Could you check a few things on this model? Use its own coordinates, in mm. A direction names the side the tool comes from. Coordinates: 2 decimals unless noted, no trailing zeros. Order: outer loops, then holes, each group sorted by start corner. A loop starts at its lowest first (then second) coordinate and runs counter-clockwise, first axis right, second up. Notation, with made-up numbers: (75.5, 87) - (123.5, 87) arc R24 ccw to (123.5, 109) - close; hole circle Ø1 at (44, 76). An arc over 180 degrees is marked (long way). Answer as a JSON object with one key per item and string values. Group by question number.
(1) We'd pull the mould along Z, two halves only. Please class faces 5 (the cylindrical face through (-0.1, -2.9, 14.5)), 6 (the flat face through (-13, -22.5, 13)), 7 (the flat face through (-8, 1, 0)): pulls with the +Z half, pulls with the -Z half, needs draft (parallel to the pull), parting line crosses it, or undercut.
(2) Will these pins go through, and if not, where does the flat tip stop? P1, Ø12, axis at x = 0, y = 30, coming from the -Z side; P2, Ø1.5, axis at y = -33, z = 14.5, coming from the -X side; P3, Ø5, axis at y = 8, z = 15.5, coming from the +X side; P4, Ø2.5, axis at x = -13.5, z = 14.5, coming from the +Y side.
(3) Imagine slicing it at B-B, the plane x = -0.75. Write out the boundary of the cut face in (y, z).
(4) Which directions (+Z, -Z, +X, -X, +Y, -Y) give clear straight access to the entire face, cutting with the end or side of a thin tool? Please do faces 1 (the flat face through (-13, 2.5, 13)), 2 (the cylindrical face through (-0.1, -2.9, 11.5)), 3 (the flat face through (6.5, -3, 7)), 4 (the cylindrical face through (-0.1, -3.1, 23.5)).
(5) Imagine slicing it at D-D, the plane z = 3.75. Write out the boundary of the cut face in (x, y).
(6) Imagine slicing it at A-A, the plane z = 13. Write out the boundary of the cut face in (x, y), and give its area (3 significant figures).
(7) Imagine slicing it at C-C, the plane y = 34. Write out the boundary of the cut face in (x, z).
(8) Please list where these lines run through material, in increasing order: probe 1 along Y at (x, z) = (0, 12.75); probe 2 along Y at (x, z) = (0, 6.5); probe 3 along Y at (x, z) = (7, 7.25).
from build123d import *

# Parameters (mm, degrees)
ESBO_O1_R                = 7.65
RESSALTO_EXTRUS_O1_DEPTH = 26
RESSALTO_EXTRUS_O2_DEPTH = 13
ESBO_O7_W                = 15
ESBO_O7_H                = 25
RESSALTO_EXTRUS_O3_DEPTH = 3
ESBO_O8_R                = 1.5
CORTE_EXTRUS_O1_DEPTH    = 15


with BuildPart() as part:
    # Esbo_o1 → Ressalto-extrus_o1 (new body)
    with BuildSketch(Plane.XY):
        with BuildLine():
            Line((-11.65, 30), (-11.65, 28))
            Line((-11.65, 28), (-11.65, -30))
            ThreePointArc((-11.65, -30), (10.282205503, -35.477111465), (-6.5, -20.331882293))
            Line((-6.5, -20.331882293), (-6.5, 20.331882293))
            ThreePointArc((-6.5, 20.331882293), (10.282205503, 35.477111465), (-11.65, 30))
        make_face()
        with Locations(Location((0, 30, 0), (0, 0, 180))):
            Circle(ESBO_O1_R, mode=Mode.SUBTRACT)
        with Locations(Location((0, -30, 0), (0, 0, 180))):
            Circle(ESBO_O1_R, mode=Mode.SUBTRACT)
    extrude(amount=RESSALTO_EXTRUS_O1_DEPTH)

    # Esbo_o6 → Ressalto-extrus_o2 (add)
    with BuildSketch(Plane(origin=(-6.5, 0, 0), x_dir=(0, 0, -1), z_dir=(1, 0, 0))):
        with BuildLine():
            Line((-17.5, -6), (-20.5, -6))
            ThreePointArc((-20.5, -6), (-23.5, -3), (-20.5, 0))
            Line((-20.5, 0), (-17.5, 0))
            ThreePointArc((-17.5, 0), (-14.5, -3), (-17.5, -6))
        make_face()
        with BuildLine():
            Line((-8.5, -6), (-5.5, -6))
            ThreePointArc((-5.5, -6), (-2.5, -3), (-5.5, 0))
            Line((-5.5, 0), (-8.5, 0))
            ThreePointArc((-8.5, 0), (-11.5, -3), (-8.5, -6))
        make_face()
    extrude(amount=RESSALTO_EXTRUS_O2_DEPTH)

    # Esbo_o7 → Ressalto-extrus_o3 (add)
    with BuildSketch(Plane.ZY.offset(11.65)):
        with Locations((13, -10)):
            Rectangle(ESBO_O7_W, ESBO_O7_H)
    extrude(amount=RESSALTO_EXTRUS_O3_DEPTH)

    # Esbo_o8 → Corte-extrus_o1 (cut)
    with BuildSketch(Plane.ZY.offset(14.65)):
        with Locations(Location((13, -10, 0), (0, 0, 270))):
            Circle(ESBO_O8_R)
    extrude(amount=-CORTE_EXTRUS_O1_DEPTH, mode=Mode.SUBTRACT)


solid = part.part
Result set:
{
 "1": {"face 5": "undercut", "face 6": "needs draft", "face 7": "pulls with the -Z half"},
 "2": {"P1": "passes through", "P2": "stops at x = -11.43", "P3": "stops at x = -6.5", "P4": "stops at y = 2.5"},
 "3": {"outline": "(-41.63, 0) - (-37.61, 0) - (-37.61, 26) - (-41.63, 26) - close; (-22.39, 0) - (-18.37, 0) - (-18.37, 26) - (-22.39, 26) - close; (-6, 5.5) arc R3 ccw to (0, 5.5) - (0, 8.5) arc R3 ccw to (-6, 8.5) - close; (-6, 17.5) arc R3 ccw to (0, 17.5) - (0, 20.5) arc R3 ccw to (-6, 20.5) - close; (18.37, 0) - (22.39, 0) - (22.39, 26) - (18.37, 26) - close; (37.61, 0) - (41.63, 0) - (41.63, 26) - (37.61, 26) - close"},
 "4": {"face 1": "+Z, -Z, -X, +Y", "face 2": "+X", "face 3": "+Z, -Z, +X", "face 4": "+Z, +X"},
 "5": {"outline": "(-11.65, -30) arc R11.65 ccw (long way) to (-6.5, -20.33) - (-6.5, -5.44) - (6.5, -5.44) - (6.5, -0.56) - (-6.5, -0.56) - (-6.5, 20.33) arc R11.65 ccw (long way) to (-11.65, 30) - close; hole circle Ø15.3 at (0, -30); hole circle Ø15.3 at (0, 30)"},
 "6": {"outline": "(-14.65, -22.5) - (-11.65, -22.5) - (-11.65, -30) arc R11.65 ccw (long way) to (-6.5, -20.33) - (-6.5, -11.5) - (-14.65, -11.5) - close; (-14.65, -8.5) - (-6.5, -8.5) - (-6.5, 20.33) arc R11.65 ccw (long way) to (-11.65, 30) - (-11.65, 2.5) - (-14.65, 2.5) - close; hole circle Ø15.3 at (0, -30); hole circle Ø15.3 at (0, 30)", "area": "775 mm^2"},
 "7": {"outline": "(-10.94, 0) - (-6.52, 0) - (-6.52, 26) - (-10.94, 26) - close; (6.52, 0) - (10.94, 0) - (10.94, 26) - (6.52, 26) - close"},
 "8": {"probe 1": "y = -41.65 to -37.65, -22.35 to -18.35, 18.35 to 22.35, 37.65 to 41.65", "probe 2": "y = -41.65 to -37.65, -22.35 to -18.35, -6 to 0, 18.35 to 22.35, 37.65 to 41.65", "probe 3": "y = -39.31 to -33.09, -26.91 to -20.69, 20.69 to 26.91, 33.09 to 39.31"}
}
